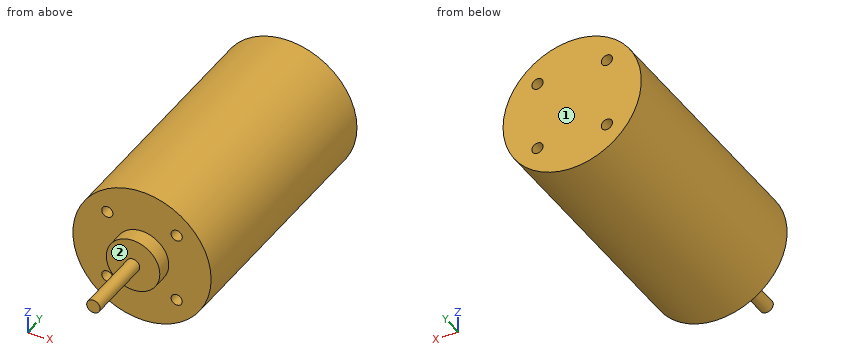
from build123d import *

# Parameters (mm, degrees)
F0_R     = 15.5
F1_DEPTH = 57
F2_R     = 6
F3_DEPTH = 3.5
F4_R     = 1.5
F5_DEPTH = 15.5
F6_D     = 2.5


with BuildPart() as f1:
    # F0 (on Front) → F1 (new body)
    with BuildSketch(Plane.XZ):
        Circle(F0_R)
    extrude(amount=F1_DEPTH)

    # F2 (on face) → F3 (join)
    with BuildSketch(Plane.XZ.offset(57)):
        Circle(F2_R)
    extrude(amount=F3_DEPTH)

    # F4 (on face) → F5 (join)
    with BuildSketch(Plane.XZ.offset(60.5)):
        Circle(F4_R)
    extrude(amount=F5_DEPTH)

    # F6 (through all)
    with Locations(Plane.XZ.offset(57)):
        with Locations((-7.7781745931, 7.7781745931), (7.7781745931, 7.7781745931), (7.7781745931, -7.7781745931), (-7.7781745931, -7.7781745931)):
            Hole(F6_D / 2)


solid = f1.part
The listing builds one solid part. Answer for the finished solid, in the listing's coordinates (mm). Face numbers are marked on the shaded views. A direction names the side the tool comes from. Coordinates: 2 decimals unless noted, no trailing zeros. Write each loop counter-clockwise with the first axis right and the second up, starting at its lowest first coordinate (ties: lowest second). Pieces come first, ordered by that corner, then holes. Notation, with made-up numbers: M 43.25,53.25 L 58.25,53.25 A6 cw 58.25,61.25 Z; hole C 64.5,-12 d9. An arc over 180 degrees is marked long. Put each result on its own line as item: value. Start each with the question number.
1. A cutting plane is placed at B-B on z = 0. Write down the section's boundary in (x, y), then the cut area to 3 significant figures.
2. A cutting plane is placed at A-A on x = 0. Write down the section's boundary in (y, z).
3. A cutting plane is placed at D-D on y = -40.5. Write down the section's boundary in (x, z).
4. Consider line 1 (X direction, y = -27, z = 7.5); line 2 (X direction, y = -34.5, z = 8). Determine where each line is inside the solid, lowest interval first. Write a range as from..to.
5. Which of the six approach directions +Z, -Z, +X, -X, +Y, -Y give full straight-line access (tool end or side, diameter ignored) to the marked faces 1 and 2?
6. A cutting plane is placed at C-C on x = 7.5. Write down the section's boundary in (y, z), then the cut area to 3 significant figures.
7. Flat-ended cylindrical pins translate along their axes: P1, Ø2, axis at x = 6.5, y = -26.5, coming from the +Z side; P2, Ø10, axis at x = -11.5, y = -52.5, coming from the +Z side; P3, Ø10, axis at x = 4.5, z = -12, coming from the -Y side. Find the tip coordinate at first contact, or state that the pin passes through.
Resolved:
1. outline: M -15.5,-57 L -6,-57 L -6,-60.5 L -1.5,-60.5 L -1.5,-76 L 1.5,-76 L 1.5,-60.5 L 6,-60.5 L 6,-57 L 15.5,-57 L 15.5,0 L -15.5,0 Z
1. area: 1,860 mm2
2. outline: M -76,-1.5 L -60.5,-1.5 L -60.5,-6 L -57,-6 L -57,-15.5 L 0,-15.5 L 0,15.5 L -57,15.5 L -57,6 L -60.5,6 L -60.5,1.5 L -76,1.5 Z
3. outline: C 0,0 d31; hole C -7.78,-7.78 d2.5; hole C -7.78,7.78 d2.5; hole C 7.78,-7.78 d2.5; hole C 7.78,7.78 d2.5
4. line 1: x = -13.56..-9, -6.56..6.56, 9..13.56
4. line 2: x = -13.28..-9.01, -6.55..6.55, 9.01..13.28
5. face 1: +Z, -Z, +X, -X, +Y
5. face 2: -Y
6. outline: M -57,-13.56 L 0,-13.56 L 0,-9 L -57,-9 Z; M -57,-6.56 L 0,-6.56 L 0,6.56 L -57,6.56 Z; M -57,9 L 0,9 L 0,13.56 L -57,13.56 Z
6. area: 1,270 mm2
7. P1: stops at z = 14.49
7. P2: stops at z = 14.07
7. P3: stops at y = -57
